Design review of the part shown in the three views and the two pictorial views. Dimensions are in mm from the part's minimum x, y and z. Round coordinates to 2 decimals unless told otherwise and drop trailing zeros. Order: outer loops, then holes, each group sorted by start corner. A loop starts at its lowest first (then second) coordinate and runs counter-clockwise, first axis right, second up. Notation, with made-up numbers: (29.5, 5) - (41.5, 5) arc R23 cw to (41.5, 24) - close; hole circle Ø9 at (-40, 30.5). An arc over 180 degrees is marked (long way). One line per question, with ' | ' between items. Start each with the question number.
Item 1: Add section A-A on z = 10. State the section outline as (x, y) points, and give its area (3 significant figures).
Item 2: Add section C-C on z = 17.25. State the section outline as (x, y) points, and give its area (3 significant figures).
Item 3: For L1, parallel to X at y = 26, z = 17.5; L2, parallel to Y at x = 138.5, z = 17.25; L3, parallel to Z at x = 70, y = 76, list the stretches that pass through material, from the lowest coordinate up. Write a range as [from, to].
Item 4: Draft analysis for pull direction X (two halves, no side actions). For the marked faces 1 and 2, state which applies: +X half, -X half, draft (parallel to the pull), parting line (faces both ways), or undercut.
Item 5: Add section B-B on x = 43. State the section outline as (y, z) points, and give its area (3 significant figures).
Item 6: Insertion check: pin 1 Ø1 at (x, y) = (61.5, 27) entering from +Z. The pin has a flat end and moves straight along its axis. Give the tip position at first contact, or say it passes through.
Item 7: Add section D-D on y = 55.5. State the section outline as (x, z) points.
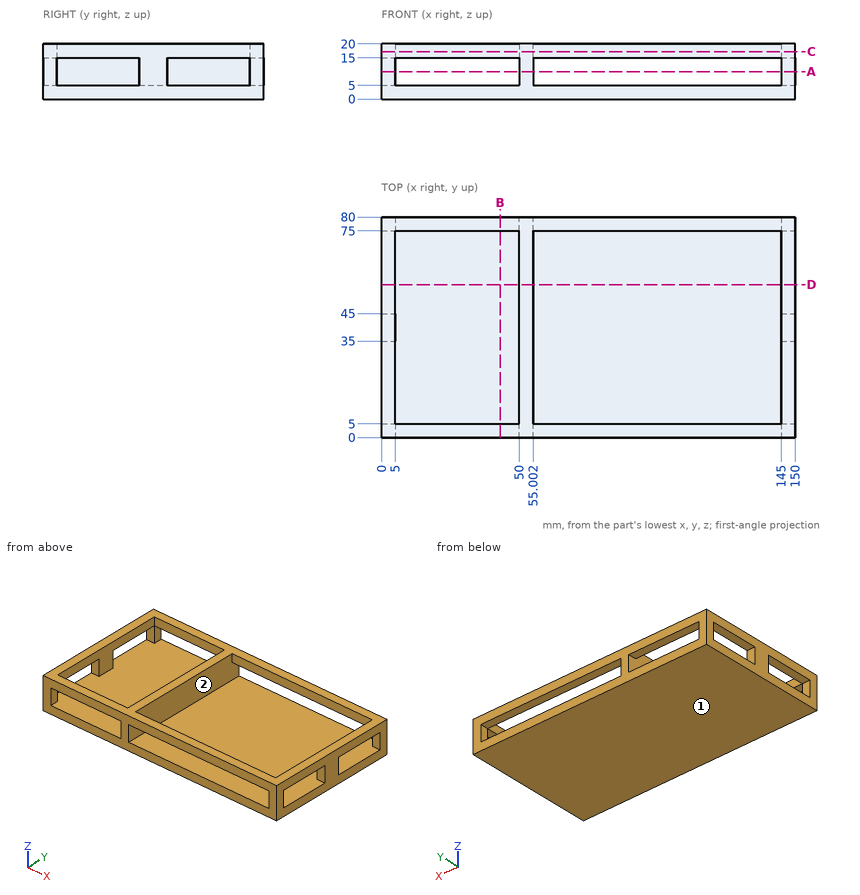
Determined:
1) outline: (0, 0) - (5, 0) - (5, 5) - (0, 5) - close; (0, 35) - (5, 35) - (5, 45) - (0, 45) - close; (0, 75) - (5, 75) - (5, 80) - (0, 80) - close; (50, 0) - (55, 0) - (55, 80) - (50, 80) - close; (145, 0) - (150, 0) - (150, 5) - (145, 5) - close; (145, 35) - (150, 35) - (150, 45) - (145, 45) - close; (145, 75) - (150, 75) - (150, 80) - (145, 80) - close | area: 600 mm2
2) outline: (0, 0) - (150, 0) - (150, 80) - (0, 80) - close; hole (5, 5) - (50, 5) - (50, 75) - (5, 75) - close; hole (55, 5) - (145, 5) - (145, 75) - (55, 75) - close | area: 2,550 mm2
3) L1: [0, 5], [50, 55], [145, 150] | L2: [0, 5], [75, 80] | L3: [0, 5], [15, 20]
4) face 1: draft | face 2: undercut
5) outline: (0, 0) - (80, 0) - (80, 5) - (0, 5) - close; (0, 15) - (5, 15) - (5, 20) - (0, 20) - close; (75, 15) - (80, 15) - (80, 20) - (75, 20) - close | area: 450 mm2
6) pin 1: z = 5
7) outline: (0, 0) - (150, 0) - (150, 5) - (55, 5) - (55, 20) - (50, 20) - (50, 5) - (0, 5) - close; (0, 15) - (5, 15) - (5, 20) - (0, 20) - close; (145, 15) - (150, 15) - (150, 20) - (145, 20) - close
